Can you work these out from the model? Positions are in its coordinate system, mm. Face numbers are marked on the shaded views. A direction names the side the tool comes from. Coordinates: 2 decimals unless noted, no trailing zeros. Answer in a Markdown table with one row per item. Add a question column.
1. Will these pins go through, and if not, where does the flat tip stop? pin 1 (1.5 mm diameter, centred on x = 1.5, y = -4, fed in from +Z); pin 2 (4 mm diameter, centred on x = 6.5, z = 9.5, fed in from -Y); pin 3 (2.5 mm diameter, centred on y = -5, z = 19, fed in from -X).
2. If I drill on line 1 along Y through (x, z) = (3, 29); line 2 along Y through (x, z) = (0.75, 30.5); line 3 along Z through (x, y) = (0, -1.25), over which ranges is the centre line in solid material (lowest first)? Write a range as [from, to].
3. We'd pull the mould along Z, two halves only. Please class the marked faces 1, 2, 3 and 4: pulls with the +Z half, pulls with the -Z half, needs draft (parallel to the pull), parting line crosses it, or undercut.
4. On a 3-axis mill with a long thin cutter (end or side, diameter ignored), from which of +Z, -Z, +X, -X, +Y, -Y can I reach the whole of each face in a straight line? I mean the marked faces 5, 6, 7 and 8. Say none if no direction works.
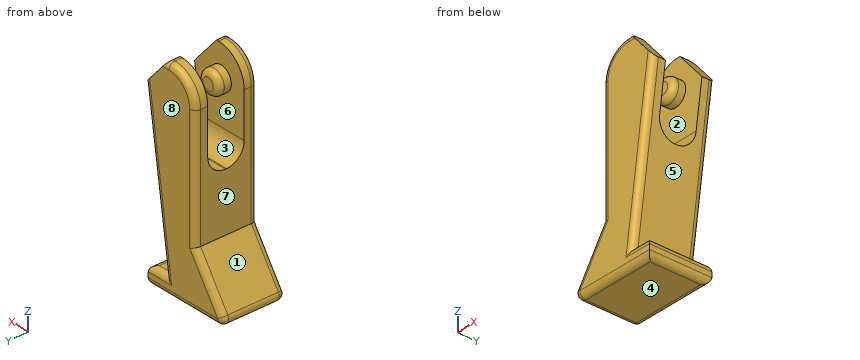
from build123d import *

# Parameters (mm, degrees)
F1_DEPTH = 10.6
F2_R     = 5
F3_SIZE  = 5
F4_W     = 6.2000000016
F4_H     = 15.6
F5_DEPTH = 12.5
F7_R     = 2
F8_DEPTH = 2.2
F10_R    = 1
F11_R    = 3


with BuildPart() as f1:
    # F0 (on Front) → F1 (new body)
    with BuildSketch(Plane.XZ):
        Polygon((-1.36, 9.4), (-7.7, 0), (7.7, 0), (7.7, 2.88), (4.3, 2.88), (9.04, 34.9), (-1.36, 34.9), align=None)
    extrude(amount=F1_DEPTH)

    # F2
    f2_edges = [f1.edges().sort_by_distance(p)[0] for p in [
        (-1.36, -5.3, 34.9),
    ]]
    fillet(f2_edges, radius=F2_R)

    # F3
    f3_edges = [f1.edges().sort_by_distance(p)[0] for p in [
        (9.04, -5.3, 34.9),
    ]]
    chamfer(f3_edges, length=F3_SIZE)

    # F4 (on Right) → F5 (cut, symmetric)
    with BuildSketch(Plane.YZ):
        with Locations((-5.2999999992, 27.100082695)):
            Rectangle(F4_W, F4_H)
    extrude(amount=F5_DEPTH, both=True, mode=Mode.SUBTRACT)

    # F7 (on face) → F8 (join)
    with BuildSketch(Plane.XZ.offset(2.1999999984)):
        with Locations((3.14, 29.6)):
            Circle(F7_R)
    extrude(amount=F8_DEPTH)

    # F9: F1 across plane


with BuildPart() as f1_1:
    add(f1.part)
    add(f1.part.mirror(Plane.XZ.offset(5.3)))

    # F10
    f10_edges = [f1_1.edges().sort_by_distance(p)[0] for p in [
        (1.14, -6.2, 29.6),
        (1.14, -4.4, 29.6),
        (-4.53, 0, 4.7),
        (-7.7, -5.3, 0),
        (-4.53, -10.6, 4.7),
        (-1.36, -10.6, 19.65),
        (-1.36, 0, 19.65),
        (6.303908, 0, 16.41695),
        (6.303908, -10.6, 16.41695),
        (6, -10.6, 2.88),
        (7.7, -5.3, 2.88),
        (6, 0, 2.88),
        (0, 0, 0),
        (7.7, -5.3, 0),
        (0, -10.6, 0),
    ]]
    fillet(f10_edges, radius=F10_R)

    # F11
    f11_edges = [f1_1.edges().sort_by_distance(p)[0] for p in [
        (2.685353, -2.2, 19.300083),
        (2.685353, -8.4, 19.300083),
    ]]
    fillet(f11_edges, radius=F11_R)


solid = f1_1.part
Answers follow:
| question | item | result |
|---|---|---|
| 1 | pin 1 | stops at z = 31.31 |
| 1 | pin 2 | stops at y = -10.58 |
| 1 | pin 3 | stops at x = -1.36 |
| 2 | line 1 | y = [-10.6, -6.2], [-4.4, 0] |
| 2 | line 2 | y = [-10.6, -8.4], [-2.2, 0] |
| 2 | line 3 | z = [0, 33.33] |
| 3 | face 1 | pulls with the +Z half |
| 3 | face 2 | undercut |
| 3 | face 3 | undercut |
| 3 | face 4 | pulls with the -Z half |
| 4 | face 5 | +X, +Y, -Y |
| 4 | face 6 | none |
| 4 | face 7 | +Z, -X, +Y, -Y |
| 4 | face 8 | +Z, -Z, +X, -X, +Y |
